from build123d import *

# Parameters (mm, degrees)
ESQUISSE1_W                = 200
ESQUISSE1_H                = 200
BOSS_EXTRU_1_DEPTH         = 6.35
BOSS_EXTRU_2_DEPTH         = 6.35
ENL_V_MAT_EXTRU_1_REACH    = 149.324
ESQUISSE3_R                = 1.5875
R_P_TITION_LIN_AIRE1_COUNT = 2
R_P_TITION_LIN_AIRE1_PITCH = 190
SYM_TRIE1_COPY_1_DEPTH     = 6.35
SYM_TRIE1_COPY_2_REACH     = 149.324
SYM_TRIE1_COPY_2_SKETCH_R  = 1.5875
ESQUISSE4_W                = 75
ESQUISSE4_H                = 50
BOSS_EXTRU_3_DEPTH         = 6.35
CONG_1_R                   = 10


with BuildPart() as part:
    # Esquisse1 → Boss.-Extru.1 (new body)
    with BuildSketch(Plane(origin=(0, 0, 0), x_dir=(1, 0, 0), z_dir=(0, 1, 0))):
        Rectangle(ESQUISSE1_W, ESQUISSE1_H)
    extrude(amount=BOSS_EXTRU_1_DEPTH)

    # Esquisse2 → Boss.-Extru.2 (add)
    with BuildSketch(Plane(origin=(0, 6.35, 0), x_dir=(1, 0, 0), z_dir=(0, 1, 0))):
        with BuildLine():
            Line((-100, 100), (-90, 100))
            Line((-90, 100), (-90, 103))
            ThreePointArc((-90, 103), (-95, 108), (-100, 103))
            Line((-100, 103), (-100, 100))
        make_face()
    boss_extru_2 = extrude(amount=-BOSS_EXTRU_2_DEPTH)

    # Esquisse3 → Enlèv. mat.-Extru.1 (cut, up to next)
    with BuildSketch(Plane(origin=(0, 6.35, 0), x_dir=(1, 0, 0), z_dir=(0, 1, 0)), mode=Mode.PRIVATE) as enl_v_mat_extru_1_sk1:
        with Locations(Location((-95, 103, 0), (0, 0, 270))):
            Circle(ESQUISSE3_R)
    enl_v_mat_extru_1_tool1 = extrude(enl_v_mat_extru_1_sk1.sketch, amount=-ENL_V_MAT_EXTRU_1_REACH, mode=Mode.PRIVATE) & part.part
    enl_v_mat_extru_1 = enl_v_mat_extru_1_tool1.solids().sort_by_distance((-95, 6.35, -103))[0]
    add(enl_v_mat_extru_1, mode=Mode.SUBTRACT)

    # Répétition linéaire1: Boss.-Extru.2, Enlèv. mat.-Extru.1 ×2
    with Locations(*[(i * R_P_TITION_LIN_AIRE1_PITCH, 0, 0) for i in range(1, R_P_TITION_LIN_AIRE1_COUNT)]):
        add(boss_extru_2)
        add(enl_v_mat_extru_1, mode=Mode.SUBTRACT)

    # Symétrie1: Boss.-Extru.2, Enlèv. mat.-Extru.1 across plane
    add(boss_extru_2.mirror(Plane.XY))
    add(enl_v_mat_extru_1.mirror(Plane.XY), mode=Mode.SUBTRACT)

    # Symétrie1 copy 1 sketch → Symétrie1 copy 1 (add)
    with BuildSketch(Plane(origin=(190, 6.35, 0), x_dir=(1, 0, 0), z_dir=(0, 1, 0))):
        with BuildLine():
            Line((-100, -100), (-90, -100))
            Line((-90, -100), (-90, -103))
            ThreePointArc((-90, -103), (-95, -108), (-100, -103))
            Line((-100, -103), (-100, -100))
        make_face()
    extrude(amount=-SYM_TRIE1_COPY_1_DEPTH)

    # Symétrie1 copy 2 sketch → Symétrie1 copy 2 (cut, up to next)
    with BuildSketch(Plane(origin=(190, 6.35, 0), x_dir=(1, 0, 0), z_dir=(0, 1, 0)), mode=Mode.PRIVATE) as sym_trie1_copy_2_sk1:
        with Locations((-95, -103)):
            Circle(SYM_TRIE1_COPY_2_SKETCH_R)
    sym_trie1_copy_2_tool1 = extrude(sym_trie1_copy_2_sk1.sketch, amount=-SYM_TRIE1_COPY_2_REACH, mode=Mode.PRIVATE) & part.part
    add(sym_trie1_copy_2_tool1.solids().sort_by_distance((95, 6.35, 103))[0], mode=Mode.SUBTRACT)

    # Esquisse4 → Boss.-Extru.3 (add)
    with BuildSketch(Plane(origin=(0, 6.35, 0), x_dir=(1, 0, 0), z_dir=(0, 1, 0))):
        with Locations((0, 125)):
            Rectangle(ESQUISSE4_W, ESQUISSE4_H)
    extrude(amount=-BOSS_EXTRU_3_DEPTH)

    # Congé1
    cong_1_edges = [part.edges().sort_by_distance(p)[0] for p in [
        (-37.5, 3.175, -150),
        (37.5, 3.175, -150),
    ]]
    fillet(cong_1_edges, radius=CONG_1_R)


solid = part.part
The listing builds one solid part. Answer for the finished solid, in the listing's coordinates (mm). A direction names the side the tool comes from. Give positions to 0.01 mm unless a question says otherwise; leave off trailing zeros. Write each loop counter-clockwise with the first axis right and the second up, starting at its lowest first coordinate (ties: lowest second). Pieces come first, ordered by that corner, then holes. Notation, with made-up numbers: (-5.5, 39.5) - (31.5, 39.5) arc R27 ccw to (31.5, 68.5) - close; hole circle Ø10 at (-38.75, -14.5). An arc over 180 degrees is marked (long way). One line per question, with ' | ' between items. Start each with the question number.
1. Determine the mould class of faces 1 (the face through (63, 3, -100)), 2 (the face through (34.65, 3.13, -146.99)), 3 (the face through (-100, 3, 1)) for opening direction X: +X half, -X half, draft (parallel to the pull), parting line (faces both ways), or undercut.
2. For faces 4 (the face through (-1, 3, 100)), 5 (the face through (-37.5, 3, -120)), 6 (the face through (0, 3, -150)), determine the directions among +Z, -Z, +X, -X, +Y, -Y from which every point of the face is accessible in a straight line to the end or side of a thin tool.
3. Section C-C, the plane x = 17.5 is taken. Determine the outline of the cut face in (y, z), then the cut area to 3 significant figures.
4. Section B-B, the plane x = 55 is taken. Determine the outline of the cut face in (y, z).
5. Given P1, Ø1.9, axis at x = 95, z = 103, coming from the +Y side; P2, Ø1.9, axis at y = 3, z = -111, coming from the -X side; P3, Ø3, axis at x = 71.5, y = 2, coming from the +Z side; P4, Ø1.9, axis at y = 3.5, z = -123.5, coming from the +X side, each flat-ended and moving along its own axis, determine where each tip first touches the part or whether it passes through.
6. Straight lines are drawn through the part: line 1 (X direction, y = 3, z = -103); line 2 (Z direction, x = 95, y = 5.25); line 3 (X direction, y = 3.25, z = 103). For each, find the intervals that lie inside material, in ascending order.
7. Section A-A, the plane y = 2.25 is taken. Determine the outline of the cut face in (x, z) (1 decimal), then the cut area to 3 significant figures.
Result:
1) face 1: undercut | face 2: +X half | face 3: -X half
2) face 4: +Z, +Y, -Y | face 5: -Z, +Y, -Y | face 6: -Z, +X, -X, +Y, -Y
3) outline: (0, -150) - (6.35, -150) - (6.35, 100) - (0, 100) - close | area: 1,590 mm2
4) outline: (0, -100) - (6.35, -100) - (6.35, 100) - (0, 100) - close
5) P1: passes through | P2: stops at x = -37.5 | P3: stops at z = 100 | P4: stops at x = 37.5
6) line 1: x = -100 to -96.59, -93.41 to -90, -37.5 to 37.5, 90 to 93.41, 96.59 to 100 | line 2: z = -108 to -104.59, -101.41 to 101.41, 104.59 to 108 | line 3: x = -100 to -96.59, -93.41 to -90, 90 to 93.41, 96.59 to 100
7) outline: (-100, -103) arc R5 ccw to (-90, -103) - (-90, -100) - (-37.5, -100) - (-37.5, -140) arc R10 ccw to (-27.5, -150) - (27.5, -150) arc R10 ccw to (37.5, -140) - (37.5, -100) - (90, -100) - (90, -103) arc R5 ccw to (100, -103) - (100, 103) arc R5 ccw to (90, 103) - (90, 100) - (-90, 100) - (-90, 103) arc R5 ccw to (-100, 103) - close; hole circle Ø3.2 at (-95, -103); hole circle Ø3.2 at (-95, 103); hole circle Ø3.2 at (95, -103); hole circle Ø3.2 at (95, 103) | area: 44,000 mm2
